```python
from build123d import *

# Parameters (mm, degrees)
PAD002_DEPTH    = 7
PAD003_DEPTH    = 3
CHAMFER003_SIZE = 1.5
SKETCH009_W     = 7.9
SKETCH009_H     = 8.3
PAD004_DEPTH    = 7.9
FILLET001_R     = 3.94
SKETCH010_R     = 1
HOLE002_DEPTH   = 25
SKETCH016_W     = 8.5
SKETCH016_H     = 7
POCKET003_DEPTH = 4
SKETCH017_W     = 8.5
SKETCH017_H     = 4
POCKET004_DEPTH = 4


with BuildPart() as part:
    # Sketch006 → Pad002 (new body)
    with BuildSketch(Plane.XY.offset(4)):
        Polygon((-62, 2.5), (-62, -16), (62, -16), (62, 2.5), (42, 2.5), (31.5, -8), (-31.5, -8), (-42, 2.5), align=None)
    extrude(amount=PAD002_DEPTH)

    # Sketch007 (on Face9 of Pad002) → Pad003 (join)
    with BuildSketch(Plane(origin=(0, 0, 4), x_dir=(1, 0, 0), z_dir=(0, 0, -1))):
        with BuildLine():
            Line((-31.5, 8), (31.5, 8))
            Line((37.293259, 2.206741), (31.5, 8))
            Line((38.566051, 3.479533), (37.293259, 2.206741))
            Line((32.772792, 9.272792), (38.566051, 3.479533))
            ThreePointArc((32.772792, 9.272792), (32.18883, 9.662983), (31.5, 9.8))
            Line((31.5, 9.8), (-31.5, 9.8))
            ThreePointArc((-31.5, 9.8), (-32.18883, 9.662983), (-32.772792, 9.272792))
            Line((-38.566051, 3.479533), (-32.772792, 9.272792))
            Line((-37.293259, 2.206741), (-38.566051, 3.479533))
            Line((-31.5, 8), (-37.293259, 2.206741))
        make_face()
    extrude(amount=PAD003_DEPTH)

    # Chamfer003
    chamfer003_edges = [part.edges().sort_by_distance(p)[0] for p in [
        (-35.669422, -6.376163, 4),
    ]]
    chamfer(chamfer003_edges, length=CHAMFER003_SIZE)

    # Sketch009 (on Face1 of Chamfer003) → Pad004 (join)
    with BuildSketch(Plane(origin=(0, 0, 4), x_dir=(1, 0, 0), z_dir=(0, 0, -1))):
        with Locations((-58.05, 6.75)):
            Rectangle(SKETCH009_W, SKETCH009_H)
    extrude(amount=PAD004_DEPTH)

    # Fillet001
    fillet001_edges = [part.edges().sort_by_distance(p)[0] for p in [
        (-54.1, -6.75, -3.9),
        (-62, -6.75, -3.9),
    ]]
    fillet(fillet001_edges, radius=FILLET001_R)

    # Sketch010 (on Face1 of Fillet001) → Hole002 (cut)
    with BuildSketch(Plane.XZ.offset(10.9)):
        with Locations((-58, 0)):
            Circle(SKETCH010_R)
    extrude(amount=-HOLE002_DEPTH, mode=Mode.SUBTRACT)

    # Sketch016 (on Face19 of Hole002) → Pocket003 (cut)
    with BuildSketch(Plane.YZ.offset(62)):
        with Locations((-6.75, 7.5)):
            Rectangle(SKETCH016_W, SKETCH016_H)
    extrude(amount=-POCKET003_DEPTH, mode=Mode.SUBTRACT)

    # Sketch017 (on Face21 of Pocket003) → Pocket004 (cut)
    with BuildSketch(Plane.YZ.offset(58)):
        with Locations((-6.75, 9)):
            Rectangle(SKETCH017_W, SKETCH017_H)
    extrude(amount=-POCKET004_DEPTH, mode=Mode.SUBTRACT)


solid = part.part
```
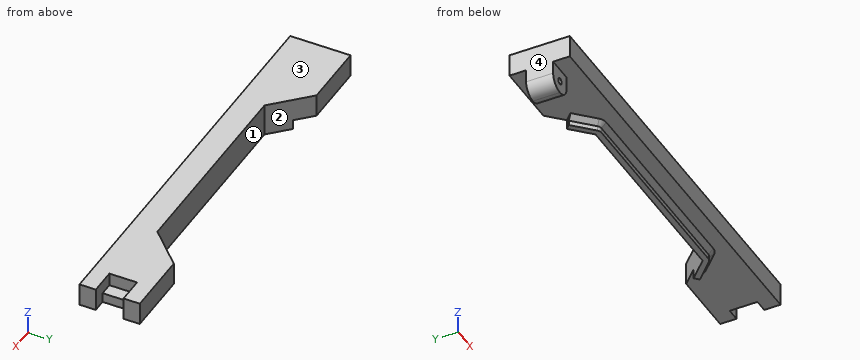
The model under review builds one solid part; all positions refer to its coordinate system, in mm. Face numbers are marked on the shaded views. Give positions to 0.01 mm unless a question says otherwise; leave off trailing zeros. Loops run counter-clockwise (first coordinate to the right, second up) from the corner with the lowest first, then second, coordinate; pieces in that order, holes last. Notation, with made-up numbers: (26, 25.5) - (42, 25.5) arc R23 ccw to (42, 33.5) - close; hole circle Ø4 at (55, -16). An arc over 180 degrees is marked (long way). Answer as a JSON object with one key per item and string values.
Q1. Add section B-B on x = -2. State the section outline as (y, z) points, plus the area to 3 significant figures.
Worked out:
{"outline": "(-16, 4) - (-11.3, 4) - (-9.8, 2.5) - (-9.8, 1) - (-8, 1) - (-8, 11) - (-16, 11) - close", "area": "62.5 mm^2"}
Q2. Add section D-D on z = -2.25. State the section outline as (x, y) points.
Worked out:
{"outline": "(-61.27, -10.9) - (-54.83, -10.9) - (-54.83, -2.6) - (-61.27, -2.6) - close"}
Q3. Mouldability with a two-part tool opening along X and no side actions: class the marked faces 1, 2, 3 and 4 as +X half, -X half, draft (parallel to the pull), parting line (faces both ways), or undercut.
Worked out:
{"face 1": "undercut", "face 2": "undercut", "face 3": "draft", "face 4": "-X half"}
Q4. Add section A-A on y = 0. State the section outline as (x, z) points, plus the area to 3 significant figures.
Worked out:
{"outline": "(-62, 4) - (-39.5, 4) - (-39.5, 11) - (-62, 11) - close; (39.5, 4) - (62, 4) - (62, 11) - (39.5, 11) - close", "area": "315 mm^2"}
Q5. Insertion check: pin 1 (1.2 mm diameter, centred on x = -5, z = 2, fed in from -Y); pin 2 (4.5 mm diameter, centred on y = -6.5, z = 1.5, fed in from +X); pin 3 (5 mm diameter, centred on x = -11, z = 4.5, fed in from +Y). Each pin has a flat end and moves straight along its axis. Give the tip position at first contact, or say it passes through.
Worked out:
{"pin 1": "stops at y = -9.9", "pin 2": "stops at x = 38.03", "pin 3": "stops at y = -8"}
Q6. Add section C-C on y = -12.5. State the section outline as (x, z) points, plus the area to 3 significant figures.
Worked out:
{"outline": "(-62, 4) - (62, 4) - (62, 11) - (-62, 11) - close", "area": "868 mm^2"}
Q7. To check wall thickness, follow line 1 along Z through (x, y) = (-58, -6.5); line 2 along Y through (x, z) = (4.5, 1.25); line 3 along Y through (x, z) = (27, 10.5). State the ranges of each line that lie inside material, in increasing order.
Worked out:
{"line 1": "z = -3.9 to -1, 1 to 11", "line 2": "y = -9.8 to -8", "line 3": "y = -16 to -8"}
